Can you work these out from the drawing? Everything is in mm from the part's minimum corner. Coordinates: 2 decimals unless noted, no trailing zeros. Write each loop counter-clockwise with the first axis right and the second up, starting at its lowest first coordinate (ties: lowest second). Pieces come first, ordered by that corner, then holes. Notation, with made-up numbers: (-35.75, 5) -> (14.25, 5) arc R27 cw to (14.25, 35) -> close; hole circle Ø10 at (70, 76.25). An arc over 180 degrees is marked (long way). Use a Markdown table: item, result. Add a question column.
Item 1: If I drill on line 1 along Z through (x, y) = (89, 2.4); line 2 along Z through (x, y) = (20, 3.55); line 3 along X through (y, z) = (3.5, 19), over which ranges is the centre line in solid material (lowest first)? Write a range as from..to.
Item 2: Imagine slicing it at A-A, the plane x = 16. Write out the boundary of the cut face in (y, z).
Item 3: Will these pins go through, and if not, where does the flat tip stop? pin 1 Ø1.5 at (x, y) = (34, 1.5) entering from +Z (3 decimals); pin 2 Ø1 at (y, z) = (1, 84) entering from +X.
Item 4: Imagine slicing it at B-B, the plane z = 88. Write out the boundary of the cut face in (x, y).
Item 5: Imagine slicing it at D-D, the plane x = 63. Write out the boundary of the cut face in (y, z), and give its area (3 significant figures).
Item 6: Imagine slicing it at C-C, the plane y = 2.85. Write out the boundary of the cut face in (x, z), and give its area (3 significant figures).
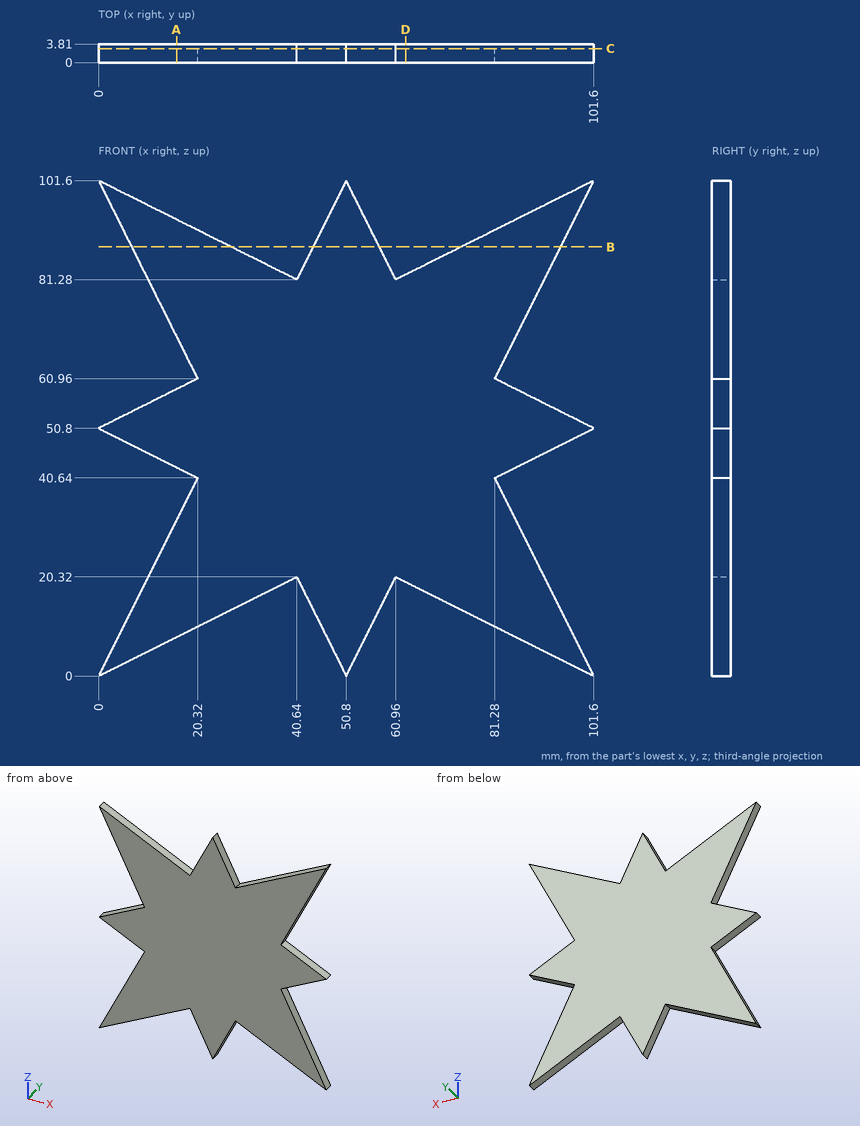
Ans:
| question | item | result |
|---|---|---|
| 1 | line 1 | z = 6.3..25.2, 44.5..57.1, 76.4..95.3 |
| 1 | line 2 | z = 10..40, 40.8..60.8, 61.6..91.6 |
| 1 | line 3 | x = 9.5..38, 41.3..60.3, 63.6..92.1 |
| 2 | outline | (0, 8) -> (3.81, 8) -> (3.81, 32) -> (0, 32) -> close; (0, 42.8) -> (3.81, 42.8) -> (3.81, 58.8) -> (0, 58.8) -> close; (0, 69.6) -> (3.81, 69.6) -> (3.81, 93.6) -> (0, 93.6) -> close |
| 3 | pin 1 | stops at z = 84.975 |
| 3 | pin 2 | stops at x = 93.05 |
| 4 | outline | (6.8, 0) -> (27.2, 0) -> (27.2, 3.81) -> (6.8, 3.81) -> close; (44, 0) -> (57.6, 0) -> (57.6, 3.81) -> (44, 3.81) -> close; (74.4, 0) -> (94.8, 0) -> (94.8, 3.81) -> (74.4, 3.81) -> close |
| 5 | outline | (0, 19.3) -> (3.81, 19.3) -> (3.81, 82.3) -> (0, 82.3) -> close |
| 5 | area | 240 mm^2 |
| 6 | outline | (0, 0) -> (40.64, 20.32) -> (50.8, 0) -> (60.96, 20.32) -> (101.6, 0) -> (81.28, 40.64) -> (101.6, 50.8) -> (81.28, 60.96) -> (101.6, 101.6) -> (60.96, 81.28) -> (50.8, 101.6) -> (40.64, 81.28) -> (0, 101.6) -> (20.32, 60.96) -> (0, 50.8) -> (20.32, 40.64) -> close |
| 6 | area | 6,190 mm^2 |
